The listing builds one solid part. Answer for the finished solid, in the listing's coordinates (mm). A direction names the side the tool comes from. Give positions to 0.01 mm unless a question says otherwise; leave off trailing zeros. Order: outer loops, then holes, each group sorted by start corner. A loop starts at its lowest first (then second) coordinate and runs counter-clockwise, first axis right, second up. Notation, with made-up numbers: (60, 65.25) - (71, 65.25) arc R27 cw to (71, 87.25) - close; hole circle Ø8 at (31, -39.5). An arc over 180 degrees is marked (long way). Answer as a JSON object with one key per item and string values. Group by question number.
Q1. A cutting plane is placed at A-A, the plane y = 28.5. Give the vertices of the cut face in (x, z).
Q2. A cutting plane is placed at C-C, the plane y = 6. Give the vertices of the cut face in (x, z), and give its area (3 significant figures).
Q3. For faces 1 (the face through (0, 0, 0)), 2 (the face through (0, 0.4, 0)), determine the directions among +Z, -Z, +X, -X, +Y, -Y from which every point of the face is accessible in a straight line to the end or side of a thin tool.
Q4. Consider line 1 (Y direction, x = 13.5, z = -3); line 2 (Z direction, x = -3, y = 30.5); line 3 (Z direction, x = -12.5, y = 5). Determine where each line is inside the solid, lowest interval first.
Q5. A cutting plane is placed at B-B, the plane z = 0. Give the vertices of the cut face in (x, y), and give its area (3 significant figures).
Q6. Given pin 1 (1.5 mm diameter, centred on x = 6, y = 20, fed in from -Z); pin 2 (4 mm diameter, centred on x = -17, y = 26.5, fed in from -Z); pin 3 (6 mm diameter, centred on y = 27, z = -11.5, fed in from -X), each flat-ended and moving along its own axis, determine where each tip first touches the part or whether it passes through.
Q7. The mould has two halves that part along X. Classify faces 3 (the face through (-13, 35, -26)), 4 (the face through (-13.68, 21.51, 23.57)): released by +X, released by -X, zero draft, split by the parting line, or undercut.
from build123d import *

# Parameters (mm, degrees)
BOSS_EXTRUDE1_DEPTH = 35
CUT_EXTRUDE2_DEPTH  = 36
BOSS_EXTRUDE2_DEPTH = 0.4
FILLET1_R           = 8


with BuildPart() as part:
    # Sketch1 → Boss-Extrude1 (new body)
    with BuildSketch(Plane(origin=(0, 0, 0), x_dir=(1, 0, 0), z_dir=(0, 1, 0))):
        with BuildLine():
            ThreePointArc((1.451818925, -34.068556857), (1.641248992, -34.346908706), (1.964225605, -34.442038138))
            ThreePointArc((1.964225605, -34.442038138), (26.591847487, -21.978073076), (34.198225299, 4.555174015))
            ThreePointArc((34.198225299, 4.555174015), (23.590291339, 25.176355888), (2.324135821, 34.423627607))
            ThreePointArc((2.324135821, 34.423627607), (1.751838249, 34.289058819), (1.354061739, 33.856153382))
            ThreePointArc((1.354061739, 33.856153382), (0, 33.001534515), (-1.354061739, 33.856153382))
            ThreePointArc((-1.354061739, 33.856153382), (-1.751838249, 34.289058819), (-2.324135821, 34.423627607))
            ThreePointArc((-2.324135821, 34.423627607), (-23.590291339, 25.176355888), (-34.198225299, 4.555174015))
            ThreePointArc((-34.198225299, 4.555174015), (-26.591847487, -21.978073076), (-1.964225605, -34.442038138))
            ThreePointArc((-1.964225605, -34.442038138), (-1.641248992, -34.346908706), (-1.451818925, -34.068556857))
            ThreePointArc((-1.451818925, -34.068556857), (0, -32.945679925), (1.451818925, -34.068556857))
        make_face()
        with BuildLine():
            Line((-2.417, 3.787737139), (0, 3.787737139))
            Line((0, 3.787737139), (2.417, 3.787737139))
            ThreePointArc((2.417, 3.787737139), (0, -4.489512172), (-2.417, 3.787737139))
        make_face(mode=Mode.SUBTRACT)
    extrude(amount=BOSS_EXTRUDE1_DEPTH)

    # Sketch2 → Cut-Extrude2 (cut, through all)
    with BuildSketch(Plane(origin=(0, 0, 0), x_dir=(1, 0, 0), z_dir=(0, 1, 0))):
        with BuildLine():
            ThreePointArc((-17.316046237, 24.498051815), (-25.980762114, 15), (-29.873958333, 2.747110027))
            ThreePointArc((-29.873958333, 2.747110027), (-27.25, 0), (-29.873958333, -2.747110027))
            ThreePointArc((-29.873958333, -2.747110027), (-25.980762114, -15), (-17.316046237, -24.498051815))
            ThreePointArc((-17.316046237, -24.498051815), (-13.625, -23.599192253), (-12.557912097, -27.245161842))
            ThreePointArc((-12.557912097, -27.245161842), (0, -30), (12.557912097, -27.245161842))
            ThreePointArc((12.557912097, -27.245161842), (13.625, -23.599192253), (17.316046237, -24.498051815))
            ThreePointArc((17.316046237, -24.498051815), (25.980762114, -15), (29.873958333, -2.747110027))
            ThreePointArc((29.873958333, -2.747110027), (27.25, 0), (29.873958333, 2.747110027))
            ThreePointArc((29.873958333, 2.747110027), (25.980762114, 15), (17.316046237, 24.498051815))
            ThreePointArc((17.316046237, 24.498051815), (13.625, 23.599192253), (12.557912097, 27.245161842))
            ThreePointArc((12.557912097, 27.245161842), (0, 30), (-12.557912097, 27.245161842))
            ThreePointArc((-12.557912097, 27.245161842), (-13.625, 23.599192253), (-17.316046237, 24.498051815))
        make_face()
    extrude(amount=CUT_EXTRUDE2_DEPTH, mode=Mode.SUBTRACT)

    # Sketch2<2> → Boss-Extrude2 (add)
    with BuildSketch(Plane(origin=(0, 0, 0), x_dir=(1, 0, 0), z_dir=(0, 1, 0))):
        with BuildLine():
            ThreePointArc((-17.316046237, 24.498051815), (-25.980762114, 15), (-29.873958333, 2.747110027))
            ThreePointArc((-29.873958333, 2.747110027), (-27.25, 0), (-29.873958333, -2.747110027))
            ThreePointArc((-29.873958333, -2.747110027), (-25.980762114, -15), (-17.316046237, -24.498051815))
            ThreePointArc((-17.316046237, -24.498051815), (-13.625, -23.599192253), (-12.557912097, -27.245161842))
            ThreePointArc((-12.557912097, -27.245161842), (0, -30), (12.557912097, -27.245161842))
            ThreePointArc((12.557912097, -27.245161842), (13.625, -23.599192253), (17.316046237, -24.498051815))
            ThreePointArc((17.316046237, -24.498051815), (25.980762114, -15), (29.873958333, -2.747110027))
            ThreePointArc((29.873958333, -2.747110027), (27.25, 0), (29.873958333, 2.747110027))
            ThreePointArc((29.873958333, 2.747110027), (25.980762114, 15), (17.316046237, 24.498051815))
            ThreePointArc((17.316046237, 24.498051815), (13.625, 23.599192253), (12.557912097, 27.245161842))
            ThreePointArc((12.557912097, 27.245161842), (0, 30), (-12.557912097, 27.245161842))
            ThreePointArc((-12.557912097, 27.245161842), (-13.625, 23.599192253), (-17.316046237, 24.498051815))
        make_face()
    extrude(amount=BOSS_EXTRUDE2_DEPTH)

    # Fillet1
    fillet1_edges = [part.edges().sort_by_distance(p)[0] for p in [
        (25.980762114, 0.4, 15),
        (27.25, 0.4, 0),
        (25.980762114, 0.4, -15),
        (13.625, 0.4, -23.599192253),
        (0, 0.4, -30),
        (-13.625, 0.4, -23.599192253),
        (-25.980762114, 0.4, -15),
        (-27.25, 0.4, 0),
        (-25.980762114, 0.4, 15),
        (-13.625, 0.4, 23.599192253),
        (0, 0.4, 30),
        (13.625, 0.4, 23.599192253),
    ]]
    fillet(fillet1_edges, radius=FILLET1_R)


solid = part.part
Reply:
{
 "1": {"outline": "(-2.32, -34.42) arc R1 ccw to (-1.35, -33.86) arc R1.5 cw to (1.35, -33.86) arc R1 ccw to (2.32, -34.42) arc R34.5 ccw to (1.96, 34.44) arc R0.5 ccw to (1.45, 34.07) arc R1.5 cw to (-1.45, 34.07) arc R0.5 ccw to (-1.96, 34.44) arc R34.5 ccw to start; hole (-29.87, -2.75) arc R30 ccw to (-17.32, -24.5) arc R2.75 cw to (-12.56, -27.25) arc R30 ccw to (12.56, -27.25) arc R2.75 cw to (17.32, -24.5) arc R30 ccw to (29.87, -2.75) arc R2.75 cw to (29.87, 2.75) arc R30 ccw to (17.32, 24.5) arc R2.75 cw to (12.56, 27.25) arc R30 ccw to (-12.56, 27.25) arc R2.75 cw to (-17.32, 24.5) arc R30 ccw to (-29.87, 2.75) arc R2.75 cw to start"},
 "2": {"outline": "(-2.32, -34.42) arc R1 ccw to (-1.35, -33.86) arc R1.5 cw to (1.35, -33.86) arc R1 ccw to (2.32, -34.42) arc R34.5 ccw to (1.96, 34.44) arc R0.5 ccw to (1.45, 34.07) arc R1.5 cw to (-1.45, 34.07) arc R0.5 ccw to (-1.96, 34.44) arc R34.5 ccw to start; hole (-29.47, -3.07) arc R29.63 ccw to (-17.4, -23.99) arc R3.12 cw to (-12.07, -27.06) arc R29.63 ccw to (12.07, -27.06) arc R3.12 cw to (17.4, -23.99) arc R29.63 ccw to (29.47, -3.07) arc R3.12 cw to (29.47, 3.07) arc R29.63 ccw to (17.4, 23.99) arc R3.12 cw to (12.07, 27.06) arc R29.63 ccw to (-12.07, 27.06) arc R3.12 cw to (-17.4, 23.99) arc R29.63 ccw to (-29.47, 3.07) arc R3.12 cw to start", "area": "1,050 mm^2"},
 "3": {"face 1": "+Z, -Z, +X, -X, -Y", "face 2": "+Y"},
 "4": {"line 1": "y = 0 to 0.4", "line 2": "z = -34.37 to -29.85, 29.85 to 34.37", "line 3": "z = -32.16 to -23.52, 23.52 to 32.15"},
 "5": {"outline": "(-34.5, 0) - (34.5, 0) - (34.5, 35) - (27.25, 35) - (27.25, 8.4) arc R8 cw to (19.25, 0.4) - (-19.25, 0.4) arc R8 cw to (-27.25, 8.4) - (-27.25, 35) - (-34.5, 35) - close", "area": "557 mm^2"},
 "6": {"pin 1": "stops at z = -34.1", "pin 2": "stops at z = -31.07", "pin 3": "stops at x = -33.44"},
 "7": {"face 3": "zero draft", "face 4": "undercut"}
}
